For this review, use the dimensioned drawing (mm, ordinates from the lowest corner) and the shaded views. Round coordinates to 2 decimals unless told otherwise and drop trailing zeros. Order: outer loops, then holes, each group sorted by start corner. A loop starts at its lowest first (then second) coordinate and runs counter-clockwise, first axis right, second up. Notation, with made-up numbers: (-40, 15.5) - (-10, 15.5) arc R25 cw to (-10, 45.5) - close; hole circle Ø11 at (29, -3). An arc over 180 degrees is marked (long way). Write each question's results on one line, items separated by ' | '. Start each with the question number.
(1) Take a section at A-A, the plane y = 57.5. Give the boundary of the cut face in (x, z), plus the area to 3 significant figures.
(2) Take a section at D-D, the plane x = 86.5. Give the boundary of the cut face in (y, z).
(3) For L1, parallel to X at y = 37.5, z = 0.25 (1 decimal); L2, parallel to X at y = 37, z = 3.55 (1 decimal); L3, parallel to Y at x = 118, z = 3.5 (1 decimal), list the stretches that pass through material, from the lowest coordinate up. Write a range as from..to.
(4) Take a section at C-C, the plane z = 2.15. Give the number of separate pieces and of enclosed holes in the cut face, plus the area to 3 significant figures.
(5) Take a section at B-B, the plane x = 45. Give the boundary of the cut face in (y, z).
(6) Insertion check: pin 1 Ø16 at (x, y) = (115, 35) entering from +Z; pin 2 Ø1 at (x, z) = (20.5, 3.5) entering from +Y; pin 3 Ø1.5 at (y, z) = (32, 3) entering from +X. Each pin has a flat end and moves straight along its axis. Give the tip position at first contact, or say it passes through.
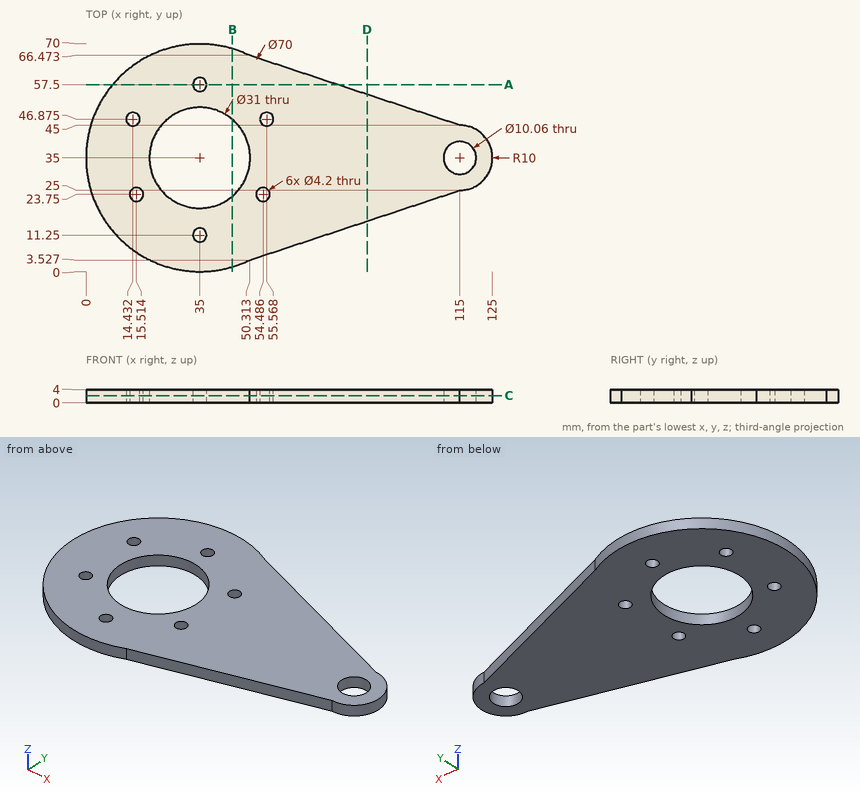
Results below:
1) outline: (8.19, 0) - (32.9, 0) - (32.9, 4) - (8.19, 4) - close; (37.1, 0) - (77.34, 0) - (77.34, 4) - (37.1, 4) - close | area: 260 mm^2
2) outline: (15.54, 0) - (54.46, 0) - (54.46, 4) - (15.54, 4) - close
3) L1: x = 0.1..19.7, 50.3..110.6, 119.4..124.7 | L2: x = 0.1..19.6, 50.4..110.4, 119.6..124.8 | L3: y = 25.5..31, 39..44.5
4) separate pieces: 1 | enclosed holes: 8 | area: 4,880 mm^2
5) outline: (1.46, 0) - (23.16, 0) - (23.16, 4) - (1.46, 4) - close; (46.84, 0) - (68.54, 0) - (68.54, 4) - (46.84, 4) - close
6) pin 1: stops at z = 4 | pin 2: stops at y = 67.08 | pin 3: stops at x = 124.74
